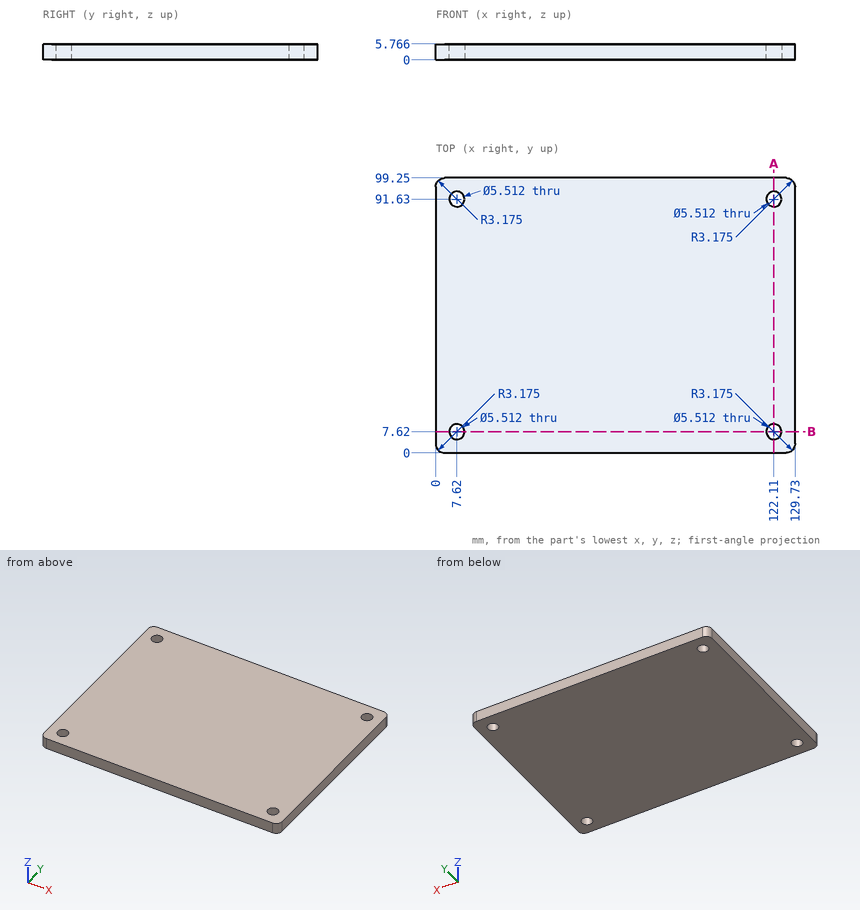
Geometry: see drawing. Coordinates: mm, zero at the bounding-box minimum. Give positions to 0.01 mm unless a question says otherwise; leave off trailing zeros. Loops run counter-clockwise (first coordinate to the right, second up) from the corner with the lowest first, then second, coordinate; pieces in that order, holes last. Notation, with made-up numbers: (-16, 57.25) -> (31, 57.25) arc R18 cw to (31, 63.25) -> close; hole circle Ø2 at (-26, 56.25). An arc over 180 degrees is marked (long way). Use one line per item in the form item = value.
Item 1: Section query A-A on x = 122.11. Output: boundary loops of the cut face in (y, z).
A:
outline = (0, 0) -> (4.86, 0) -> (4.86, 5.77) -> (0, 5.77) -> close; (10.38, 0) -> (88.87, 0) -> (88.87, 5.77) -> (10.38, 5.77) -> close; (94.39, 0) -> (99.25, 0) -> (99.25, 5.77) -> (94.39, 5.77) -> close
Item 2: Pin query (flat end, axial travel): P1, Ø6.5, axis at x = 122.11, y = 7.62, coming from the -Z side; P2, Ø4.5, axis at x = 122.11, y = 91.63, coming from the +Z side. Return the tip coordinate at first contact, or that it passes through.
A:
P1 = 0
P2 = through
Item 3: Line query: probe 1 along Y at (x, z) = (7.62, 4.35); probe 2 along Y at (x, z) = (8, 1.7). Output: solid intervals per line, ascending.
A:
probe_1 = 0 to 4.86, 10.38 to 88.87, 94.39 to 99.25
probe_2 = 0 to 4.89, 10.35 to 88.9, 94.36 to 99.25
Item 4: Section query B-B on y = 7.62. Output: boundary loops of the cut face in (x, z).
A:
outline = (0, 0) -> (4.86, 0) -> (4.86, 5.77) -> (0, 5.77) -> close; (10.38, 0) -> (119.35, 0) -> (119.35, 5.77) -> (10.38, 5.77) -> close; (124.87, 0) -> (129.73, 0) -> (129.73, 5.77) -> (124.87, 5.77) -> close
